Work out the finished part from the listing and answer in its coordinate system (mm). Face numbers are marked on the shaded views. A direction names the side the tool comes from. Coordinates: 2 decimals unless noted, no trailing zeros. Write each loop counter-clockwise with the first axis right and the second up, starting at its lowest first coordinate (ties: lowest second). Pieces come first, ordered by that corner, then holes. Notation, with made-up numbers: (-30.75, 66.25) - (-8.75, 66.25) arc R10 ccw to (-8.75, 78.25) - close; hole circle Ø7 at (34, 52). An arc over 180 degrees is marked (long way). Use one line per item in the form item = value. Start each with the question number.
Item 1: Given pin 1 (2 mm diameter, centred on x = 4, z = -1, fed in from +Y); pin 2 (2 mm diameter, centred on x = -2, z = 2, fed in from +Y), each flat-ended and moving along its own axis, determine where each tip first touches the part or whether it passes through.
Item 2: A cutting plane is placed at A-A (z = 0). Write down the section's boundary in (x, y), then the cut area to 3 significant figures.
Item 3: A cutting plane is placed at B-B (x = 1). Write down the section's boundary in (y, z).
Item 4: Determine the mould class of the marked faces 4, 5 and 6 for opening direction Z: released by +Z, released by -Z, zero draft, split by the parting line, or undercut.
Item 5: For the marked faces 1, 2 and 3, determine the directions among +Z, -Z, +X, -X, +Y, -Y from which every point of the face is accessible in a straight line to the end or side of a thin tool.
Item 6: Consider probe 1 along X at (y, z) = (0.1, 1.6); probe 2 along Y at (x, z) = (-2.25, 0.9); probe 3 along X at (y, z) = (0.6, -0.5). Determine where each line is inside the solid, lowest interval first.
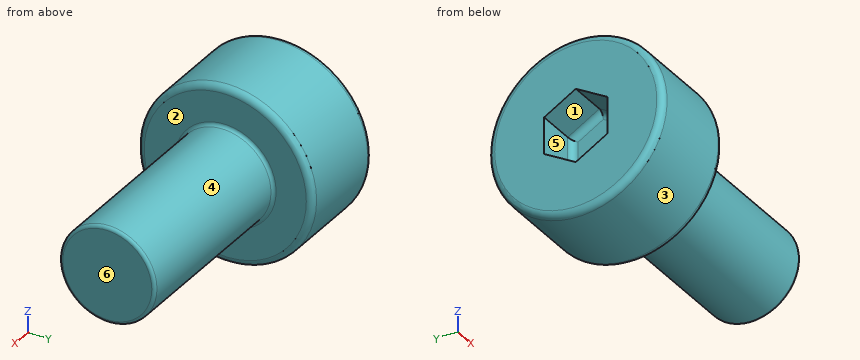
Autodesk Inventor part; units mm, degrees
ref_plane "YZ Plane" through (0, 0, 0) normal (1, 0, 0) x (0, 1, 0)
ref_plane "XZ Plane" through (0, 0, 0) normal (0, 1, 0) x (-1, 0, 0)
ref_plane "XY Plane" through (0, 0, 0) normal (0, 0, 1) x (1, 0, 0)
sketch "スケッチ1" plane through (0, 0, 0) normal (0, 0, 1) x (1, 0, 0)
  line L0 (0, 0) -> (6, 0)
  line L1 (6, 0) -> (6, 1.5)
  line L2 (6, 1.5) -> (0, 1.5)
  line L3 (0, 1.5) -> (0, 0)
  line L4 (0, 0) -> (0, 2.75)
  line L5 (0, 0) -> (-3, 0)
  line L6 (-3, 0) -> (0, 0)
  line L7 (-3, 0) -> (-3, 1.15)
  line L8 (0, 0) -> (-3, 0)
  line L9 (-3, 0) -> (-3, 2.75)
  line L10 (-3, 2.75) -> (0, 2.75)
  line L11 (0, 2.75) -> (0, 0)
  dimension "d0" = 1.5
  dimension "d1" = 6
  dimension "d3" = 3
  dimension "d4" = 2.75
  dimension "d5" = 1.15
revolve "回転1" add sketch "スケッチ1" angle 360 about axis through (-3, 0, 0) along (1, 0, 0)
thread "ねじ1"
sketch "スケッチ2" plane through (-3, 0, 0) normal (-1, 0, 0) x (0, 0, 1)
  circle A0 centre (0, 0) radius 1.15
  line L0 (-0.575, 0.9959) -> (0.575, 0.9959)
  line L1 (0.575, 0.9959) -> (1.15, 0)
  line L2 (1.15, 0) -> (0.575, -0.9959)
  line L3 (0.575, -0.9959) -> (-0.575, -0.9959)
  line L4 (-0.575, -0.9959) -> (-1.15, 0)
  line L5 (-1.15, 0) -> (-0.575, 0.9959)
  dimension "d10" = 1.15
  dimension "d11" = 1.9919
extrude "押し出し1" cut sketch "スケッチ2" against normal blind 1.4 contours L2 L3 L4 L5 L0 L1
fillet "フィレット1" radius 0.2 8 edges at (-1.6, 0.9959, 0) (-1.6, 0.498, 0.8625) (-1.6, 0.498, -0.8625) (-1.6, -0.498, -0.8625) (-1.6, -0.9959, 0) (-1.6, -0.498, 0.8625) (-3, -2.75, 0) (0, -2.75, 0)
fillet "フィレット2" radius 0.1 1 edges at (0, -1.5, 0)
fillet "フィレット3" radius 0.1 1 edges at (6, -1.5, 0)
properties part number "ネジアルミM3L6" material "アルミニウム 7075"
Answer:
q1.pin_1 = 1.5
q1.pin_2 = 2.56
q2.outline = (-3, -2.55) arc R0.2 ccw to (-2.8, -2.75) - (-0.2, -2.75) arc R0.2 ccw to (0, -2.55) - (0, -1.6) arc R0.1 cw to (0.1, -1.5) - (5.9, -1.5) arc R0.1 ccw to (6, -1.4) - (6, 1.4) arc R0.1 ccw to (5.9, 1.5) - (0.1, 1.5) arc R0.1 cw to (0, 1.6) - (0, 2.55) arc R0.2 ccw to (-0.2, 2.75) - (-2.8, 2.75) arc R0.2 ccw to (-3, 2.55) - (-3, 1) - (-1.8, 1) arc R0.2 cw to (-1.6, 0.8) - (-1.6, -0.8) arc R0.2 cw to (-1.8, -1) - (-3, -1) - close
q2.area = 31.7 mm²
q3.outline = circle Ø3 at (0, 0)
q4.face_4 = split by the parting line
q4.face_5 = undercut
q4.face_6 = zero draft
q5.face_1 = -X
q5.face_2 = +X
q5.face_3 = +X, -X
q6.probe_1 = -3 to 0
q6.probe_2 = -2.6 to -0.43, 0.43 to 2.6
q6.probe_3 = -1.6 to 6
